from build123d import *

# Parameters (mm, degrees)
BOX001_W      = 10
BOX001_H      = 10
BOX001_DEPTH  = 8
EXTRUDE_DEPTH = 10
BOX_W         = 16
BOX_H         = 16
BOX_DEPTH     = 10


with BuildPart() as cube001:
    # Box001 → Box001 (new body)
    with BuildSketch(Plane(origin=(-5, -5, 0), x_dir=(1, 0, 0), z_dir=(0, 0, 1))):
        with Locations((5, 5)):
            Rectangle(BOX001_W, BOX001_H)
    extrude(amount=BOX001_DEPTH)


with BuildPart() as extrude_body:
    # Sketch → Extrude (new body)
    with BuildSketch(Plane.XY):
        Polygon((-3.5, 0), (-1.75, -3.031089), (1.75, -3.031089), (3.5, 0), (1.75, 3.031089), (-1.75, 3.031089), align=None)
    extrude(amount=EXTRUDE_DEPTH)


with BuildPart() as extrude_body_1:
    # Extrude placement: moved
    add(extrude_body.part.moved(Location((0, 0, 10))))


with BuildPart() as cut:
    # Box → Box (new body)
    with BuildSketch(Plane(origin=(-8, -8, 0), x_dir=(1, 0, 0), z_dir=(0, 0, 1))):
        with Locations((8, 8)):
            Rectangle(BOX_W, BOX_H)
    extrude(amount=BOX_DEPTH)

    # Fusion: union Extrude body
    add(extrude_body_1.part)

    # Cut: cut Cube001
    add(cube001.part, mode=Mode.SUBTRACT)


solid = cut.part
The model under review builds one solid part; all positions refer to its coordinate system, in mm. A direction names the side the tool comes from. Coordinates: 2 decimals unless noted, no trailing zeros. Write each loop counter-clockwise with the first axis right and the second up, starting at its lowest first coordinate (ties: lowest second). Pieces come first, ordered by that corner, then holes. Notation, with made-up numbers: M 23,-8 L 46,-8 A4 ccw 46,-4 Z; hole C 47.25,41.25 d7. An arc over 180 degrees is marked long. Put each result on its own line as item: value.
1) Add section D-D on y = -2.5. Give the boundary of the cut face in (x, z), then the cut area to 3 significant figures.
Computed:
outline: M -8,0 L -5,0 L -5,8 L 5,8 L 5,0 L 8,0 L 8,10 L 2.06,10 L 2.06,20 L -2.06,20 L -2.06,10 L -8,10 Z
area: 121 mm2
2) For faces 4 (the flat face through (0, 3.031, 15)), 5 (the flat face through (0, -5, 4)), 6 (the flat face through (2.64, 1.49, 14.93)), 7 (the flat face through (0, -3.031, 15)), 8 (the flat face through (-4, 0, 10)), list the 3-axis set-ups (+Z, -Z, +X, -X, +Y, -Y) from which the entire face can be reached by the end or side of a thin tool; tool diameter is ignored.
Computed:
face 4: +Z, +X, -X, +Y
face 5: -Z
face 6: +Z, +X, +Y
face 7: +Z, +X, -X, -Y
face 8: +Z
3) Draft analysis for pull direction X (two halves, no side actions). For faces 1 (the flat face through (2.61, -1.54, 14.93)), 2 (the flat face through (0, 5, 4)), 3 (the flat face through (0, 0, 20)), state which applies: released by +X, released by -X, zero draft, split by the parting line, or undercut.
Computed:
face 1: released by +X
face 2: undercut
face 3: zero draft
4) Clearance check with flat-ended pins moving along their axes: pin 1 Ø8 at (x, y) = (0.5, -0.5) entering from -Z; pin 2 Ø4 at (x, z) = (0, 12.5) entering from -Y; pin 3 Ø3 at (x, z) = (0.5, 17.5) entering from +Y. State where each tip first meets the part, or that it passes through.
Computed:
pin 1: stops at z = 8
pin 2: stops at y = -3.03
pin 3: stops at y = 3.03
5) Add section A-A on z = 2. Give the boundary of the cut face in (x, y).
Computed:
outline: M -8,-8 L 8,-8 L 8,8 L -8,8 Z; hole M -5,-5 L 5,-5 L 5,5 L -5,5 Z
6) Wall thickness on probe 1 along X at (y, z) = (-3, 2.5); probe 2 along Z at (x, y) = (3.25, -4.75); probe 3 along Z at (x, y) = (-6.75, 0): over which ranges is each line inside the solid? List them lowest first. Write a range as [from, to].
Computed:
probe 1: x = [-8, -5], [5, 8]
probe 2: z = [8, 10]
probe 3: z = [0, 10]
7) Add section B-B on x = 4.75. Give the boundary of the cut face in (y, z).
Computed:
outline: M -8,0 L -5,0 L -5,8 L 5,8 L 5,0 L 8,0 L 8,10 L -8,10 Z
8) Add section C-C on z = 11.25. Give the boundary of the cut face in (x, y), then the cut area to 3 significant figures.
Computed:
outline: M -3.5,0 L -1.75,-3.03 L 1.75,-3.03 L 3.5,0 L 1.75,3.03 L -1.75,3.03 Z
area: 31.8 mm2
